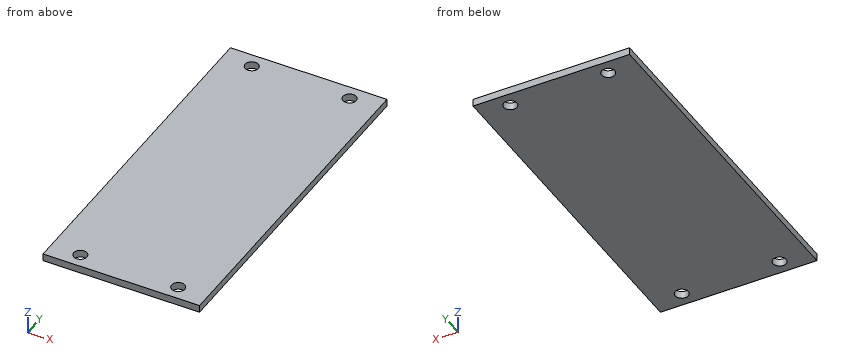
from build123d import *

# Parameters (mm, degrees)
SKETCH1_W           = 64
SKETCH1_H           = 140
SKETCH1_R           = 2.699339217
SKETCH1_W_2         = 52
SKETCH1_H_2         = 110
BOSS_EXTRUDE1_DEPTH = 3


with BuildPart() as part:
    # Sketch1 → Boss-Extrude1 (new body)
    # profile 1 of 2: a face of its own
    with BuildSketch(Plane.XY):
        with Locations((26, -55)):
            Rectangle(SKETCH1_W, SKETCH1_H)
        with Locations((46, 9)):
            Circle(SKETCH1_R, mode=Mode.SUBTRACT)
        with Locations((6, 9)):
            Circle(SKETCH1_R, mode=Mode.SUBTRACT)
        with Locations((46, -119)):
            Circle(SKETCH1_R, mode=Mode.SUBTRACT)
        with Locations((6, -119)):
            Circle(SKETCH1_R, mode=Mode.SUBTRACT)
        with Locations((26, -55)):
            Rectangle(SKETCH1_W_2, SKETCH1_H_2, mode=Mode.SUBTRACT)
    # profile 2 of 2: a face of its own
    with BuildSketch(Plane.XY):
        with Locations((26, -55)):
            Rectangle(SKETCH1_W_2, SKETCH1_H_2)
    extrude(amount=BOSS_EXTRUDE1_DEPTH)


solid = part.part
Here's how the part is built. I have some questions about the finished solid (model axes, mm). Coordinates: 2 decimals unless noted, no trailing zeros. Write each loop counter-clockwise with the first axis right and the second up, starting at its lowest first coordinate (ties: lowest second). Pieces come first, ordered by that corner, then holes.
Item 1: I want a section at A-A on y = 9. Write out the boundary of the cut face in (x, z).
Item 2: Will this pin go through, and if not, where does the flat tip stop? pin 1 (6 mm diameter, centred on x = 46, y = 9, fed in from +Z).
Item 3: If I drill on line 1 (Y direction, x = 46, z = 1); line 2 (Y direction, x = 7.5, z = 1.5), over which ranges is the centre line in solid material (lowest first)?
Item 4: I want a section at B-B on x = 6. Write out the boundary of the cut face in (y, z), and give its area (3 significant figures).
Findings below:
1. outline: (-6, 0) - (3.3, 0) - (3.3, 3) - (-6, 3) - close; (8.7, 0) - (43.3, 0) - (43.3, 3) - (8.7, 3) - close; (48.7, 0) - (58, 0) - (58, 3) - (48.7, 3) - close
2. pin 1: stops at z = 3
3. line 1: y = -125 to -121.7, -116.3 to 6.3, 11.7 to 15
3. line 2: y = -125 to -121.24, -116.76 to 6.76, 11.24 to 15
4. outline: (-125, 0) - (-121.7, 0) - (-121.7, 3) - (-125, 3) - close; (-116.3, 0) - (6.3, 0) - (6.3, 3) - (-116.3, 3) - close; (11.7, 0) - (15, 0) - (15, 3) - (11.7, 3) - close
4. area: 388 mm2
